The figure shows three views and two pictorial views of one solid part (mm, origin at its lowest corner). Answer the questions. A direction names the side the tool comes from. Round coordinates to 2 decimals unless told otherwise and drop trailing zeros. Write each loop counter-clockwise with the first axis right and the second up, starting at its lowest first coordinate (ties: lowest second). Pieces come first, ordered by that corner, then holes.
Item 1: For a pull along Z with two mould halves and no side action, classify the marked faces 1, 2 and 3 as +Z half, -Z half, draft (parallel to the pull), parting line (faces both ways), or undercut.
Item 2: Find section C-C on x = 127. Give the number of separate pieces and of enclosed holes in the cut face, then the cut area to 3 significant figures.
Item 3: Find the intervals of material crossed by probe 1 along Y at (x, z) = (209, 90); probe 2 along X at (y, z) = (102, 146) (1 decimal); probe 3 along Y at (x, z) = (64.5, 82) (1 decimal), in increasing order.
Item 4: A tool of negligible diameter and unlimited length cuts with its end or side. For the marked faces 4 and 5, from which of +Z, -Z, +X, -X, +Y, -Y can it reach the whole face along a straight path? Write none if from no direction.
Item 5: Find section D-D on y = 146.5. Give the vertices of the cut face in (x, z).
Item 6: Find section B-B on z = 19.05. Give the vertices of the cut face in (x, y), then the cut area to 3 significant figures.
Item 7: Find section A-A on z = 127. Give the vertices of the cut face in (x, y).
Item 8: Each of these flat-tipped pins is pushed along its axis until it touches: pin 1 (10 mm diameter, centred on x = 174, y = 47, fed in from -Z); pin 2 (1.5 mm diameter, centred on y = 60.5, z = 147.5, fed in from -X); pin 3 (6 mm diameter, centred on y = 183, z = 146.5, fed in from -X). Where does it stop, or does it pass through?
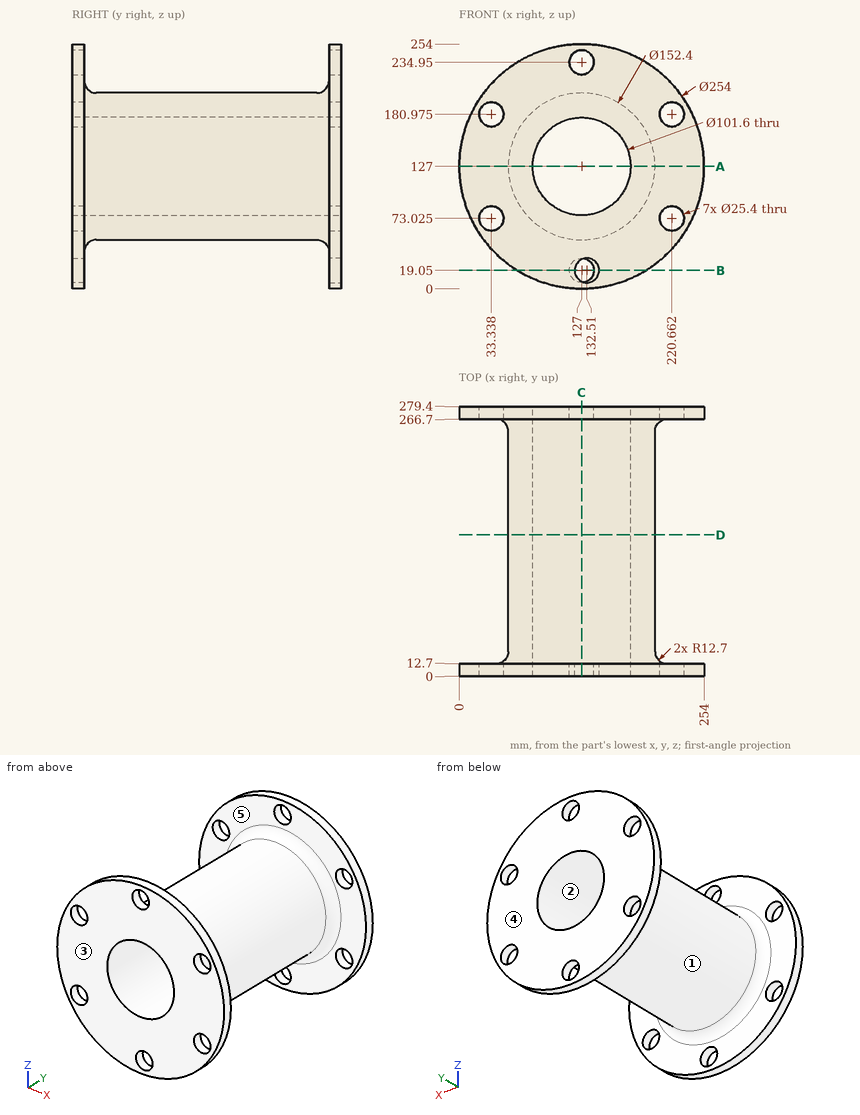
Check values:
1. face 1: parting line
1. face 2: undercut
1. face 3: draft
2. separate pieces: 6
2. enclosed holes: 0
2. area: 15,700 mm2
3. probe 1: y = 0 to 12.7, 266.7 to 279.4
3. probe 2: x = 53.2 to 79.9, 174.1 to 200.8
3. probe 3: y = 0 to 20.9, 258.5 to 279.4
4. face 4: +Z, -Z, +X, -X, +Y
4. face 5: none
5. outline: circle Ø152.4 at (127, 127); hole circle Ø101.6 at (127, 127)
6. outline: (60.1, 0) - (119.81, 0) - (119.81, 12.7) - (60.1, 12.7) - close; (60.1, 266.7) - (114.3, 266.7) - (114.3, 279.4) - (60.1, 279.4) - close; (139.7, 266.7) - (193.9, 266.7) - (193.9, 279.4) - (139.7, 279.4) - close; (145.21, 0) - (193.9, 0) - (193.9, 12.7) - (145.21, 12.7) - close
6. area: 2,750 mm2
7. outline: (0, 0) - (76.2, 0) - (76.2, 279.4) - (0, 279.4) - (0, 266.7) - (38.1, 266.7) arc R12.7 cw to (50.8, 254) - (50.8, 25.4) arc R12.7 cw to (38.1, 12.7) - (0, 12.7) - close; (177.8, 0) - (254, 0) - (254, 12.7) - (215.9, 12.7) arc R12.7 cw to (203.2, 25.4) - (203.2, 254) arc R12.7 cw to (215.9, 266.7) - (254, 266.7) - (254, 279.4) - (177.8, 279.4) - close
8. pin 1: stops at z = 63.42
8. pin 2: stops at x = 53.4
8. pin 3: stops at x = 52.61
